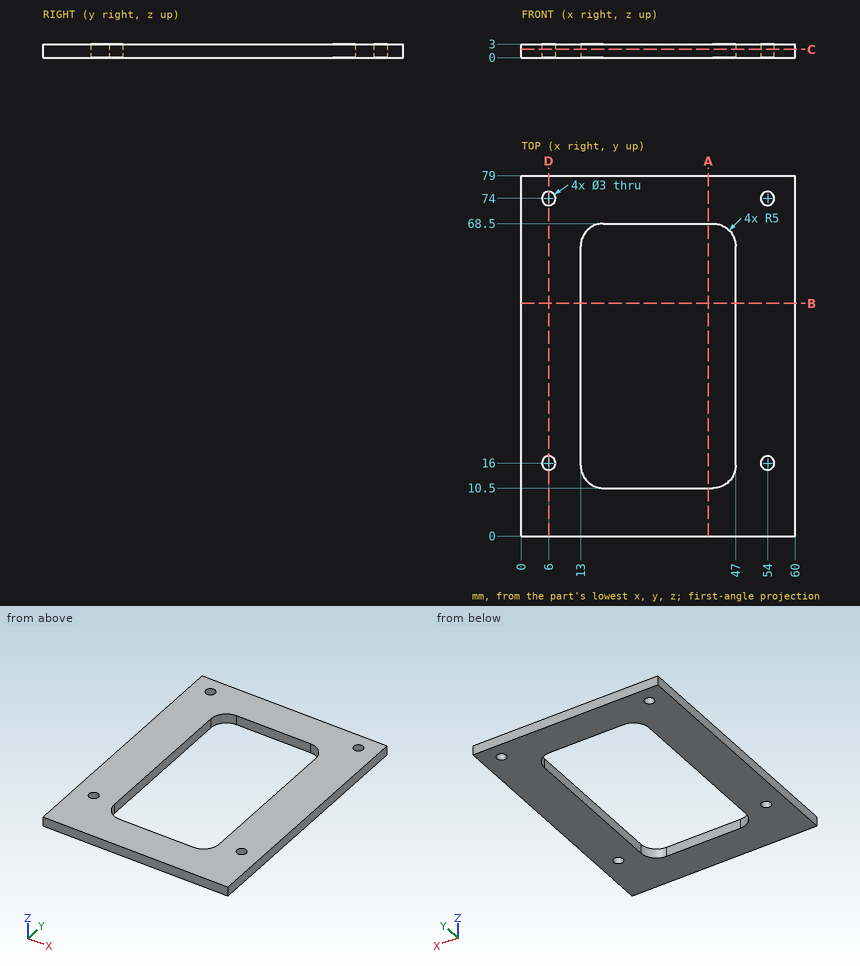
Source: three-view drawing plus pictorial views. Frame: mm from the lowest corner of the part. Give positions to 0.01 mm unless a question says otherwise; leave off trailing zeros. Order: outer loops, then holes, each group sorted by start corner. A loop starts at its lowest first (then second) coordinate and runs counter-clockwise, first axis right, second up.
1. Section B-B on y = 51. Return the cut outline in (x, z).
Derived:
outline: (0, 0) - (13, 0) - (13, 3) - (0, 3) - close; (47, 0) - (60, 0) - (60, 3) - (47, 3) - close
2. Material intervals for L1, parallel to Y at x = 54, z = 2.25; L2, parallel to X at y = 74, z = 1.6; L3, parallel to Y at x = 29, z = 2.5, sorted ascending.
Derived:
L1: y = 0 to 14.5, 17.5 to 72.5, 75.5 to 79
L2: x = 0 to 4.5, 7.5 to 52.5, 55.5 to 60
L3: y = 0 to 10.5, 68.5 to 79
3. Section A-A on x = 41. Return the cut outline in (y, z), and give its area (3 significant figures).
Derived:
outline: (0, 0) - (10.5, 0) - (10.5, 3) - (0, 3) - close; (68.5, 0) - (79, 0) - (79, 3) - (68.5, 3) - close
area: 63.0 mm2
4. Section D-D on x = 6. Return the cut outline in (y, z), and give its area (3 significant figures).
Derived:
outline: (0, 0) - (14.5, 0) - (14.5, 3) - (0, 3) - close; (17.5, 0) - (72.5, 0) - (72.5, 3) - (17.5, 3) - close; (75.5, 0) - (79, 0) - (79, 3) - (75.5, 3) - close
area: 219 mm2
5. Section C-C on z = 1.8. Return the cut outline in (x, y).
Derived:
outline: (0, 0) - (60, 0) - (60, 79) - (0, 79) - close; hole circle Ø3 at (6, 16); hole circle Ø3 at (6, 74); hole (13, 15.5) arc R5 ccw to (18, 10.5) - (42, 10.5) arc R5 ccw to (47, 15.5) - (47, 63.5) arc R5 ccw to (42, 68.5) - (18, 68.5) arc R5 ccw to (13, 63.5) - close; hole circle Ø3 at (54, 16); hole circle Ø3 at (54, 74)
